Can you work these out from the model? Positions are in its coordinate system, mm. Face numbers are marked on the shaded views. A direction names the side the tool comes from. Give positions to 0.01 mm unless a question says otherwise; leave off trailing zeros. Order: outer loops, then holes, each group sorted by start corner. A loop starts at its lowest first (then second) coordinate and runs counter-clockwise, first axis right, second up. Notation, with made-up numbers: (-11, -32) - (13, -32) arc R28 ccw to (13, -10) - close; hole circle Ø6 at (-30.5, -25.75). An arc over 180 degrees is marked (long way). Return JSON: item names as keys, results as strings.
```python
from build123d import *

# Parameters (mm, degrees)
F0_W         = 79.6983499915
F0_H         = 74.7635825602
F0_R         = 12.7
F0_H_2       = 17.6352638877
F1_DEPTH     = 25.4
F2_DEPTH     = 35.56
F4_DEPTH     = 17.6362638877
F5_R         = 12.7
F6_R         = 5.08
F7_T1_DEPTH  = 69.5383499915
F7_S5_W      = 5.08
F7_S5_H      = 5.08
F7_T6_DEPTH  = 5.08
F7_S11_W     = 5.08
F7_S11_H     = 5.08
F7_T12_DEPTH = 5.08
F8_DEPTH     = 3.048
F9_T2_ANGLE  = 250.1291990291
F9_T4_ANGLE  = 294.7758439205


# Not quite as in the source:
# - a fillet or chamfer that OpenCascade refuses, or shapes differently, is made with other operations: its cross-section is extruded or revolved along the edge and cut away or added


with BuildPart() as f1:
    # F0 (on Front) → F1 (new body)
    with BuildSketch(Plane.XZ):
        with Locations((-2.3253131658, 16.0799051921)):
            Rectangle(F0_W, F0_H)
        with Locations((0, 31.3866536387)):
            Circle(F0_R, mode=Mode.SUBTRACT)
        with Locations((-2.3253131658, -30.1195180319)):
            Rectangle(F0_W, F0_H_2)
    extrude(amount=F1_DEPTH)

    # F0 (on Front) → F2 (join)
    with BuildSketch(Plane.XZ):
        with Locations((-2.3253131658, -30.1195180319)):
            Rectangle(F0_W, F0_H_2)
    extrude(amount=-F2_DEPTH)

    # F3 (on face) → F4 (cut, through all)
    with BuildSketch(Plane.XY.offset(-21.3018860881)):
        with BuildLine():
            ThreePointArc((-12.7, 35.56), (0, 22.86), (12.7, 35.56))
            Line((12.7, 35.56), (-12.7, 35.56))
        make_face()
    extrude(amount=-F4_DEPTH, mode=Mode.SUBTRACT)

    # F5
    f5_edges = [f1.edges().sort_by_distance(p)[0] for p in [
        (-42.174488, -12.7, 53.461696),
        (37.523862, -12.7, 53.461696),
    ]]
    fillet(f5_edges, radius=F5_R)

    # F6
    f6_edges = [f1.edges().sort_by_distance(p)[0] for p in [
        (-2.325313, 0, 53.461696),
        (-2.325313, -25.4, 53.461696),
        (-42.174488, 0, 9.729905),
        (37.523862, 0, 9.729905),
        (-2.325313, 0, -21.301886),
        (37.523862, 17.78, -21.301886),
        (-42.174488, 17.78, -21.301886),
        (-42.174488, -25.4, 0.912273),
        (-42.174488, 5.08, -38.93715),
        (37.523862, -25.4, 0.912273),
        (37.523862, 5.08, -38.93715),
    ]]
    fillet(f6_edges, radius=F6_R)

    # F7: fillet of radius 5.08 on 1 edges, made by hand

    # F7_s2 → F7_t1 (cut)
    with BuildSketch(Plane.YZ.offset(-37.0944881615)):
        with BuildLine():
            ThreePointArc((-25.4, -33.8571499758), (-23.9121024484, -37.4492524242), (-20.32, -38.9371499758))
            Line((-20.32, -38.9371499758), (-25.4, -38.9371499758))
            Line((-25.4, -38.9371499758), (-25.4, -33.8571499758))
        make_face()
    extrude(amount=F7_T1_DEPTH, mode=Mode.SUBTRACT)


with BuildPart() as f7_tool4:
    # F7_s5 → F7_t6 (new body)
    with BuildSketch(Plane.XZ.offset(20.32)):
        with Locations((-39.6344881615, -36.3971499758)):
            Rectangle(F7_S5_W, F7_S5_H)
    extrude(amount=F7_T6_DEPTH)

    # F7_s7 → F7_t8 (revolve, cut)
    with BuildSketch(Plane(origin=(-37.0944881615, -20.32, -33.8571499758), x_dir=(0.7071067812, 0, 0.7071067812), z_dir=(0.7071067812, 0, -0.7071067812))):
        with BuildLine():
            ThreePointArc((0, -5.08), (5.08, 0), (0, 5.08))
            Line((0, 5.08), (0, -5.08))
        make_face()
    revolve(axis=Axis((-37.0944881615, -20.32, -33.8571499758), (0, -1, 0)), mode=Mode.SUBTRACT)


with BuildPart() as f1_1:
    add(f1.part)

    # F7_t3: cut F7_tool4
    add(f7_tool4.part, mode=Mode.SUBTRACT)


with BuildPart() as f7_tool10:
    # F7_s11 → F7_t12 (new body)
    with BuildSketch(Plane.XZ.offset(20.32)):
        with Locations((34.98386183, -36.3971499758)):
            Rectangle(F7_S11_W, F7_S11_H)
    extrude(amount=F7_T12_DEPTH)

    # F7_s13 → F7_t14 (revolve, cut)
    with BuildSketch(Plane(origin=(32.44386183, -20.32, -33.8571499758), x_dir=(-0.7071067812, 0, 0.7071067812), z_dir=(0.7071067812, 0, 0.7071067812))):
        with BuildLine():
            ThreePointArc((0, -5.08), (5.08, 0), (0, 5.08))
            Line((0, 5.08), (0, -5.08))
        make_face()
    revolve(axis=Axis((32.44386183, -20.32, -33.8571499758), (0, -1, 0)), mode=Mode.SUBTRACT)


with BuildPart() as f1_2:
    add(f1_1.part)

    # F7_t9: cut F7_tool10
    add(f7_tool10.part, mode=Mode.SUBTRACT)

    # F3 (on face) → F8 (join)
    with BuildSketch(Plane.XY.offset(-21.3018860881)):
        with BuildLine():
            Line((19.05, 35.56), (12.7, 35.56))
            ThreePointArc((12.7, 35.56), (0, 22.86), (-12.7, 35.56))
            Line((-12.7, 35.56), (-19.05, 35.56))
            ThreePointArc((-19.05, 35.56), (0, 16.51), (19.05, 35.56))
        make_face()
    extrude(amount=F8_DEPTH)

    # F9: fillet of radius 5.08 on 2 edges, made by hand

    # F9_s1 → F9_t2 (revolve, cut)
    with BuildSketch(Plane(origin=(16.7214049162, 23.823427639, 0), x_dir=(0, 0, 1), z_dir=(0.5744996444, 0.8185048311, 0))):
        with BuildLine():
            ThreePointArc((-21.3018860881, -39.4792073551), (-19.0836531533, -37.6057410411), (-18.2538860881, -34.823310449))
            Line((-18.2538860881, -34.823310449), (-18.2538860881, -39.4792073551))
            Line((-18.2538860881, -39.4792073551), (-21.3018860881, -39.4792073551))
        make_face()
    revolve(axis=Axis((0, 35.56, -18.2538860881), (0, 0, 1)), revolution_arc=F9_T2_ANGLE, mode=Mode.SUBTRACT)

    # F9_s3 → F9_t4 (revolve, cut)
    with BuildSketch(Plane(origin=(-16.14342639, 10.3289474307, 0), x_dir=(0, 0, 1), z_dir=(-0.8423388046, 0.5389483633, 0))):
        with BuildLine():
            ThreePointArc((-18.2538860881, 47.7335678904), (-19.7417836396, 44.141465442), (-23.3338860881, 42.6535678904))
            Line((-23.3338860881, 42.6535678904), (-18.2538860881, 42.6535678904))
            Line((-18.2538860881, 42.6535678904), (-18.2538860881, 47.7335678904))
        make_face()
    revolve(axis=Axis((0, 35.56, -18.2538860881), (0, 0, -1)), revolution_arc=F9_T4_ANGLE, mode=Mode.SUBTRACT)


solid = f1_2.part
```
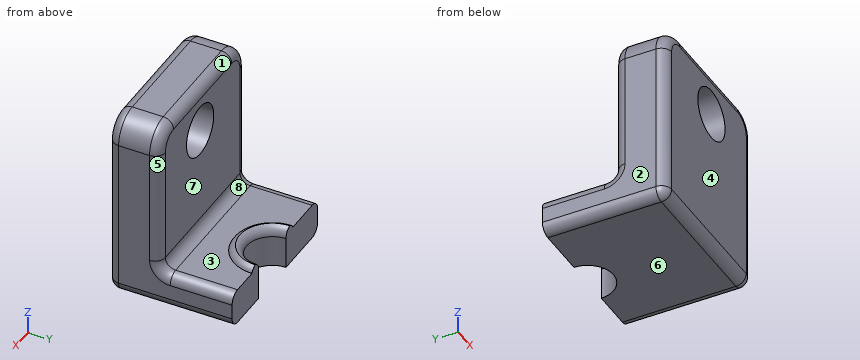
1. On a 3-axis mill with a long thin cutter (end or side, diameter ignored), from which of +Z, -Z, +X, -X, +Y, -Y can I reach the whole of each face in a straight line? I mean the marked faces 5, 6, 7 and 8. Say none if no direction works.
Checks:
{"face 5": "+Z, +X, +Y", "face 6": "-Z, +X, -X, +Y, -Y", "face 7": "+Z, +X, -X, +Y", "face 8": "+Z, +X, -X"}
2. Suppose I cut it at A-A (x = 0). List the corners of the cut face in (y, z) for me.
Checks:
{"outline": "(-25.4, -33.86) arc R5.08 ccw to (-20.32, -38.94) - (22.86, -38.94) - (22.86, -23.33) arc R5.08 ccw to (19.47, -18.54) arc R5.08 ccw to (16.51, -21.3) - (5.08, -21.3) arc R5.08 cw to (0, -16.22) - (0, 18.69) - (-25.4, 18.69) - close; (-25.4, 44.09) - (0, 44.09) - (0, 48.38) arc R5.08 ccw to (-5.08, 53.46) - (-20.32, 53.46) arc R5.08 ccw to (-25.4, 48.38) - close"}
3. If I drill on L1, parallel to Z at x = 0, y = -10; L2, parallel to Z at x = -24, y = 21; L3, parallel to Y at x = 22, z = 38, over which ranges is the centre line in solid material (lowest first)? Write a range as [from, to].
Checks:
{"L1": "[-38.94, 18.69], [44.09, 53.46]", "L2": "[-38.94, -21.3]", "L3": "[-25.4, 0]"}
4. Thinking about a two-plate mould opening in Y: for the marked faces 1, 2, 3 and 4, which applies, +Y half, -Y half, draft (parallel to the pull), parting line (faces both ways), or undercut?
Checks:
{"face 1": "+Y half", "face 2": "draft", "face 3": "undercut", "face 4": "-Y half"}
5. For pin 1 Ø9 at (x, y) = (-11.5, 22.5) entering from +Z; pin 2 Ø10 at (y, z) = (3.5, -11) entering from -X; pin 3 Ø20.5 at (x, z) = (0, 31.39) entering from -Y; pin 4 Ø12 at (x, z) = (-15, 23) entering from +Y, each with a flat end and sliding along its axis, tell me the tip position at first contact or that it passes through.
Checks:
{"pin 1": "z = -18.54", "pin 2": "x = -40.7", "pin 3": "through", "pin 4": "y = 0"}
6. Suppose I cut it at D-D (z = 27). List the corners of the cut face in (x, y) for me, plus the area to 3 significant figures.
Checks:
{"outline": "(-42.17, -20.32) arc R5.08 ccw to (-37.09, -25.4) - (-11.92, -25.4) - (-11.92, 0) - (-37.09, 0) arc R5.08 ccw to (-42.17, -5.08) - close; (11.92, -25.4) - (32.44, -25.4) arc R5.08 ccw to (37.52, -20.32) - (37.52, -5.08) arc R5.08 ccw to (32.44, 0) - (11.92, 0) - close", "area": "1,400 mm^2"}
7. Suppose I cut it at B-B (z = 3). List the corners of the cut face in (x, y) for me.
Checks:
{"outline": "(-42.17, -20.32) arc R5.08 ccw to (-37.09, -25.4) - (32.44, -25.4) arc R5.08 ccw to (37.52, -20.32) - (37.52, -5.08) arc R5.08 ccw to (32.44, 0) - (-37.09, 0) arc R5.08 ccw to (-42.17, -5.08) - close"}
8. Suppose I cut it at C-C (y = -15.5). List the corners of the cut face in (x, z) for me, plus the area to 3 significant figures.
Checks:
{"outline": "(-42.17, -33.86) arc R5.08 ccw to (-37.09, -38.94) - (32.44, -38.94) arc R5.08 ccw to (37.52, -33.86) - (37.52, 40.76) arc R12.7 ccw to (24.82, 53.46) - (-29.47, 53.46) arc R12.7 ccw to (-42.17, 40.76) - close; hole circle Ø25.4 at (0, 31.39)", "area": "6,780 mm^2"}
